from build123d import *

# Parameters (mm, degrees)
ESQUISSE10_R                       = 100
ESQUISSE10_R_2                     = 57.65
BOSS_EXTRU_1_DEPTH                 = 2
ENL_V_MAT_EXTRU_3_DEPTH            = 3
CONG_3_R                           = 8
CONG_4_R                           = 2
R_P_TITION_CIRCULAIRE4_COUNT       = 12
CONG_3_OF_R_P_TITION_CIRCULAIRE4_R = 8
CONG_4_OF_R_P_TITION_CIRCULAIRE4_R = 2


with BuildPart() as part:
    # Esquisse10 → Boss.-Extru.1 (new body, symmetric)
    with BuildSketch(Plane(origin=(0, 0, 0), x_dir=(0, 0, -1), z_dir=(1, 0, 0))):
        Circle(ESQUISSE10_R)
        Circle(ESQUISSE10_R_2, mode=Mode.SUBTRACT)
    extrude(amount=BOSS_EXTRU_1_DEPTH, both=True)

    # Esquisse11 → Enlèv. mat.-Extru.3 (cut, symmetric)
    with BuildSketch(Plane(origin=(0, 0, 0), x_dir=(0, 0, -1), z_dir=(1, 0, 0))):
        Polygon((-467.515801905, 332.57037408), (-45.619089874, 88.988193819), (0, 62.65), (0, 100), (0, 587.164360523), (-465.974399707, 1442.842054211), (-933.490201612, 1188.248067768), align=None)
    enl_v_mat_extru_3 = extrude(amount=ENL_V_MAT_EXTRU_3_DEPTH, both=True, mode=Mode.SUBTRACT)

    # Congé3
    cong_3_edges = [part.edges().sort_by_distance(p)[0] for p in [
        (0, 88.988193819, 45.619089874),
    ]]
    fillet(cong_3_edges, radius=CONG_3_R)

    # Congé4
    cong_4_edges = [part.edges().sort_by_distance(p)[0] for p in [
        (0, 62.65, 0),
    ]]
    fillet(cong_4_edges, radius=CONG_4_R)

    # Répétition circulaire4: Enlèv. mat.-Extru.3 ×12 about axis
    r_p_tition_circulaire4_axis = Axis((0, 0, 0), (1, 0, 0))
    for i in range(1, R_P_TITION_CIRCULAIRE4_COUNT):
        add(enl_v_mat_extru_3.rotate(r_p_tition_circulaire4_axis, i * 360 / R_P_TITION_CIRCULAIRE4_COUNT), mode=Mode.SUBTRACT)

    # Congé3 of Répétition circulaire4
    cong_3_of_r_p_tition_circulaire4_edges = [part.edges().sort_by_distance(p)[0] for p in [
        (0, 54.256491547, 84.001387637),
        (0, 4.986806181, 99.875581421),
        (0, -45.619089874, 88.988193819),
        (0, -84.001387637, 54.256491547),
        (0, -99.875581421, 4.986806181),
        (0, -88.988193819, -45.619089874),
        (0, -54.256491547, -84.001387637),
        (0, -4.986806181, -99.875581421),
        (0, 45.619089874, -88.988193819),
        (0, 84.001387637, -54.256491547),
        (0, 99.875581421, -4.986806181),
    ]]
    fillet(cong_3_of_r_p_tition_circulaire4_edges, radius=CONG_3_OF_R_P_TITION_CIRCULAIRE4_R)

    # Congé4 of Répétition circulaire4
    cong_4_of_r_p_tition_circulaire4_edges = [part.edges().sort_by_distance(p)[0] for p in [
        (0, 54.256491547, 31.325),
        (0, 31.325, 54.256491547),
        (0, 0, 62.65),
        (0, -31.325, 54.256491547),
        (0, -54.256491547, 31.325),
        (0, -62.65, 0),
        (0, -54.256491547, -31.325),
        (0, -31.325, -54.256491547),
        (0, 0, -62.65),
        (0, 31.325, -54.256491547),
        (0, 54.256491547, -31.325),
    ]]
    fillet(cong_4_of_r_p_tition_circulaire4_edges, radius=CONG_4_OF_R_P_TITION_CIRCULAIRE4_R)


solid = part.part
Build history of the part. All positions in model axes, mm. A direction names the side the tool comes from. Coordinates: 2 decimals unless noted, no trailing zeros. Order: outer loops, then holes, each group sorted by start corner. A loop starts at its lowest first (then second) coordinate and runs counter-clockwise, first axis right, second up. Notation, with made-up numbers: (89, 3) -> (117, 3) arc R12 ccw to (117, 7) -> close; hole circle Ø4 at (47.5, -17.75). An arc over 180 degrees is marked (long way). One line per item, written item: value.
(1) Drop flat-ended pins along their axis: pin 1 Ø2 at (x, z) = (0, 54.5) entering from +Y; pin 2 Ø1 at (x, y) = (1, 32.5) entering from +Z; pin 3 Ø2 at (x, y) = (0, 63) entering from -Z. Give the stop position or say it passes through.
Checked values:
pin 1: y = 54.26
pin 2: z = 57.16
pin 3: z = -54.26
(2) Mould opens along Z. For faces 1 (the flat face through (0.03, -76.9, 18.25)), 2 (the flat face through (0.028, 71.724, 41.41)), 3 (the flat face through (0.03, -18.25, -76.9)) say: pulls with the +Z half, pulls with the -Z half, needs draft (parallel to the pull), parting line crosses it, or undercut.
Checked values:
face 1: undercut
face 2: pulls with the +Z half
face 3: pulls with the -Z half
(3) Tool access for faces 4 (the flat face through (0.028, -41.41, 71.724)), 5 (the flat face through (2, -37, 45)), 6 (the flat face through (0.03, 18.25, 76.9)), 7 (the flat face through (0.028, -41.41, -71.724)), 8 (the flat face through (0.028, 41.41, -71.724)): list every direction of +Z, -Z, +X, -X, +Y, -Y with a clear straight run to the whole face (end or side of a thin tool).
Checked values:
face 4: +X, -X, -Y
face 5: +Z, -Z, +X, +Y, -Y
face 6: +Z, +X, -X
face 7: -Z, +X, -X
face 8: +X, -X, +Y
(4) Slice it at A-A, the plane y = 21.5. List the corners of the cut face in (x, z), plus the area to 3 significant figures.
Checked values:
outline: (-2, -75.06) -> (2, -75.06) -> (2, -53.49) -> (-2, -53.49) -> close; (-2, 53.49) -> (2, 53.49) -> (2, 71.27) -> (-2, 71.27) -> close
area: 157 mm2
(5) Probe line 1 (Z direction, x = 0.1, y = 65); line 2 (Z direction, x = -1.55, y = -85.5); line 3 (Y direction, x = -0.45, z = -83.5). List the from-to ranges inside material, lowest first. Write a range as [from, to].
Checked values:
line 1: [-54.26, -37.53], [-25.12, 0.34], [4.07, 37.53]
line 2: [-49.36, -39.58], [0, 13.29], [49.36, 51.58]
line 3: [-53.2, -48.21], [-14.44, 0], [36.11, 48.21]
